The drawing under review shows one solid part. Ordinate dimensions are in mm from its lowest x, y, z. A direction names the side the tool comes from. Coordinates: 2 decimals unless noted, no trailing zeros. Loops run counter-clockwise (first coordinate to the right, second up) from the corner with the lowest first, then second, coordinate; pieces in that order, holes last. Notation, with made-up numbers: M -19.75,-8 L 16.25,-8 A22 ccw 16.25,13 Z; hole C -14,-32 d3. An arc over 180 degrees is marked long. Put each result on its own line as item: value.
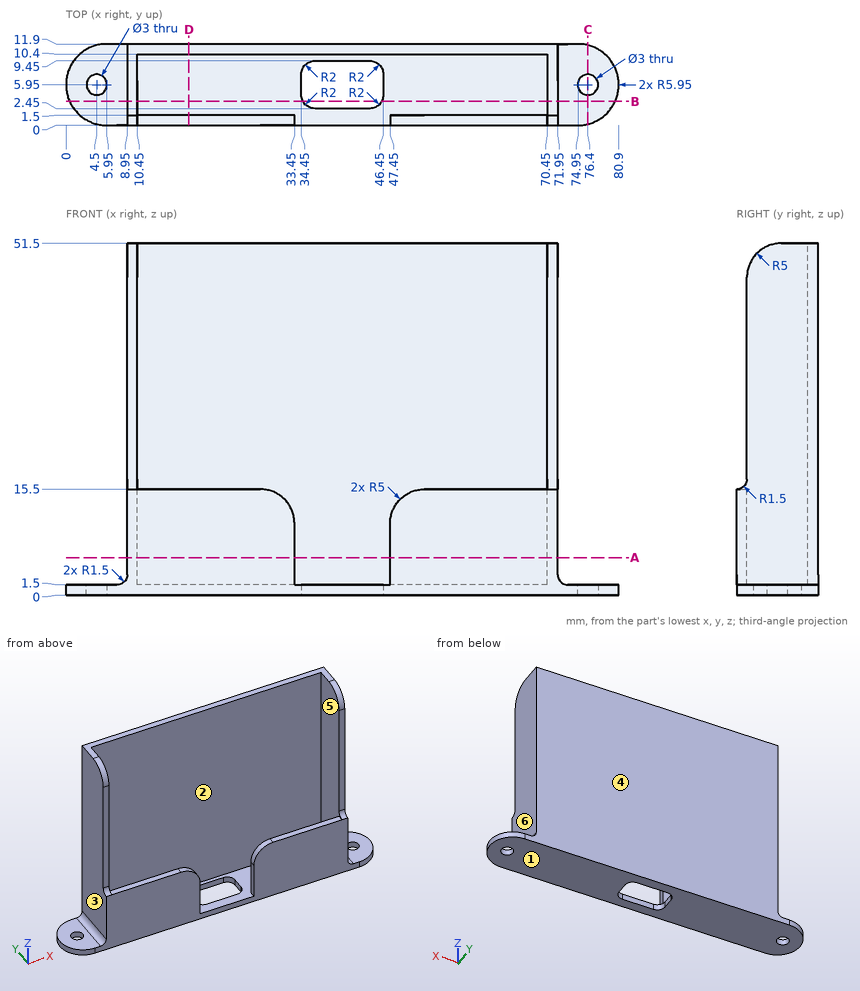
(1) Wall thickness on line 1 along Y through (x, z) = (49, 9.5); line 2 along X through (y, z) = (3.25, 19); line 3 along Z through (x, y) = (65.5, 1.75): over which ranges is each line inside the solid? List them lowest first. Write a range as [from, to].
Determined:
line 1: y = [0, 1.5], [10.4, 11.9]
line 2: x = [8.95, 10.45], [70.45, 71.95]
line 3: z = [0, 1.5]
(2) Tool access review of the marked faces 1 and 2: name each direction out of +Z, -Z, +X, -X, +Y, -Y from which nothing blocks a thin tool from reaching the whole face with its end or side.
Determined:
face 1: -Z, +X, -X, +Y, -Y
face 2: +Z
(3) Add section D-D (x = 18). Write out the cut boundary in (y, z).
Determined:
outline: M 0,0 L 11.9,0 L 11.9,51.5 L 10.4,51.5 L 10.4,1.5 L 1.5,1.5 L 1.5,15.5 L 0,15.5 Z
(4) Add section A-A (z = 5.5). Write out the cut boundary in (x, y), plus the area to 3 significant figures.
Determined:
outline: M 8.95,0 L 33.45,0 L 33.45,1.5 L 10.45,1.5 L 10.45,10.4 L 70.45,10.4 L 70.45,1.5 L 47.45,1.5 L 47.45,0 L 71.95,0 L 71.95,11.9 L 8.95,11.9 Z
area: 195 mm^2
(5) For pin 1 (1.5 mm diameter, centred on x = 21, z = 26.5, fed in from -Y); pin 2 (4 mm diameter, centred on y = 4.5, z = 28.5, fed in from +X); pin 3 (1.6 mm diameter, centred on x = 10, z = 31, fed in from -Y), all flat-tipped, find the tip position at first contact; note any pin that passes through.
Determined:
pin 1: stops at y = 10.4
pin 2: stops at x = 71.95
pin 3: stops at y = 1.5
(6) Add section B-B (y = 3.5). Write out the cut boundary in (x, z), plus the area to 3 significant figures.
Determined:
outline: M 0.53,0 L 34.69,0 L 34.69,1.5 L 10.45,1.5 L 10.45,50.5 L 8.95,50.5 L 8.95,3 A1.5 cw 7.45,1.5 L 0.53,1.5 Z; M 46.21,0 L 80.37,0 L 80.37,1.5 L 73.45,1.5 A1.5 cw 71.95,3 L 71.95,50.5 L 70.45,50.5 L 70.45,1.5 L 46.21,1.5 Z
area: 250 mm^2
(7) Draft analysis for pull direction X (two halves, no side actions). For the marked faces 3, 4, 5 and 6, state which applies: +X half, -X half, draft (parallel to the pull), parting line (faces both ways), or undercut.
Determined:
face 3: -X half
face 4: draft
face 5: undercut
face 6: +X half
(8) Add section C-C (x = 76.4). Write out the cut boundary in (y, z).
Determined:
outline: M 0.18,0 L 4.45,0 L 4.45,1.5 L 0.18,1.5 Z; M 7.45,0 L 11.72,0 L 11.72,1.5 L 7.45,1.5 Z
